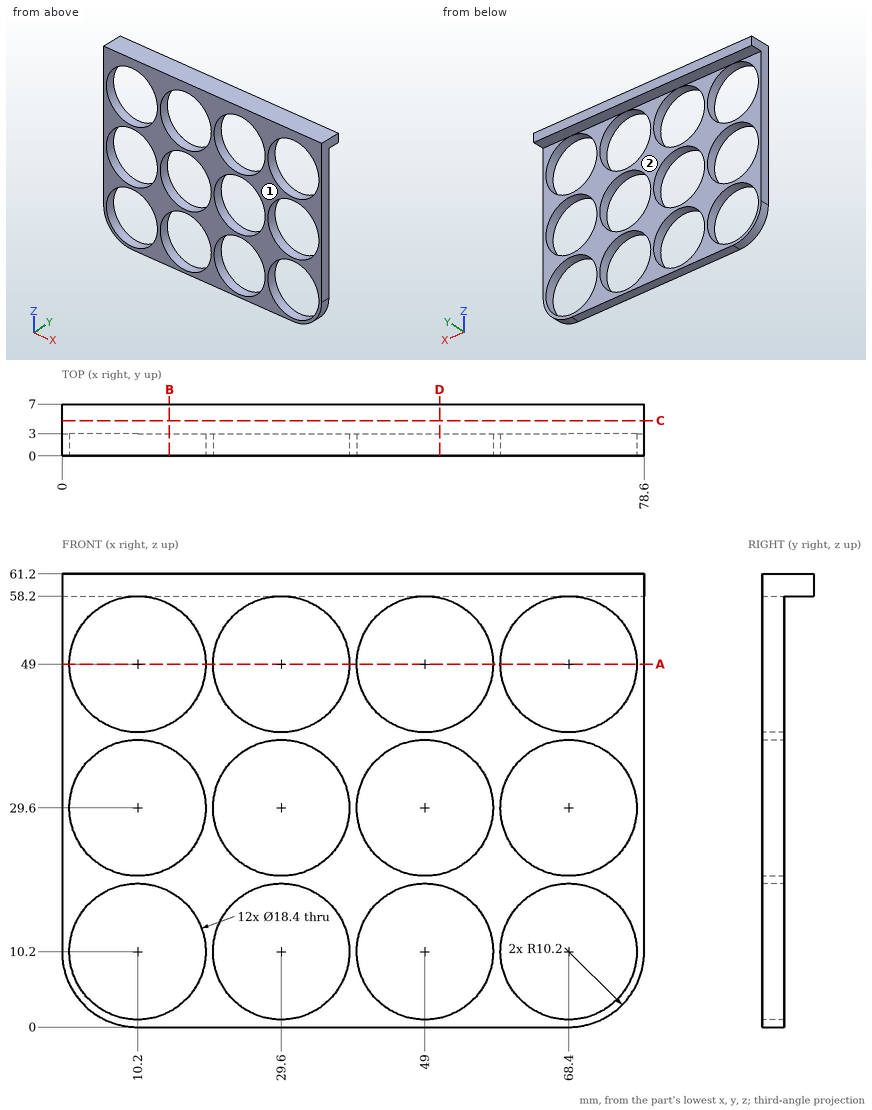
The drawing under review shows one solid part. Ordinate dimensions are in mm from its lowest x, y, z. A direction names the side the tool comes from. Give positions to 0.01 mm unless a question says otherwise; leave off trailing zeros. Order: outer loops, then holes, each group sorted by start corner. A loop starts at its lowest first (then second) coordinate and runs counter-clockwise, first axis right, second up. Notation, with made-up numbers: M 80.25,76 L 110.25,76 A21 ccw 110.25,83 Z; hole C -21,54.5 d8. An arc over 180 degrees is marked long. Answer in a Markdown table with one row per item. Add a question column.
1. Add section D-D on x = 51. State the section outline as (y, z) points.
2. For pin 1 Ø24 at (x, z) = (29.6, 10.2) entering from +Y; pin 2 Ø16.5 at (x, z) = (49, 29.6) entering from +Y; pin 3 Ø1.2 at (x, y) = (29.5, 6) entering from -Z, all flat-tipped, find the tip position at first contact; note any pin that passes through.
3. To check wall thickness, follow line 1 along X through (y, z) = (1.55, 29.6); line 2 along Z through (x, y) = (50, 2.5); line 3 along Z through (x, y) = (16, 4.5). State the ranges of each line that lie inside material, in increasing order.
4. Add section C-C on y = 4.75. State the section outline as (x, z) points, plus the area to 3 significant figures.
5. Machinability: for the marked faces 1 and 2, which of the approach directions +Z, -Z, +X, -X, +Y, -Y give a long, thin tool a straight path to every point of the face, cutting with its end or side? Answer none if there is none.
6. Add section B-B on x = 14.5. State the section outline as (y, z) points, plus the area to 3 significant figures.
7. Add section A-A on z = 49. State the section outline as (x, y) points.
The answers:
| question | item | result |
|---|---|---|
| 1 | outline | M 0,0 L 3,0 L 3,1.22 L 0,1.22 Z; M 0,19.18 L 3,19.18 L 3,20.62 L 0,20.62 Z; M 0,38.58 L 3,38.58 L 3,40.02 L 0,40.02 Z; M 0,57.98 L 3,57.98 L 3,58.2 L 7,58.2 L 7,61.2 L 0,61.2 Z |
| 2 | pin 1 | y = 3 |
| 2 | pin 2 | through |
| 2 | pin 3 | z = 58.2 |
| 3 | line 1 | 0 to 1, 19.4 to 20.4, 38.8 to 39.8, 58.2 to 59.2, 77.6 to 78.6 |
| 3 | line 2 | 0 to 1.05, 19.35 to 20.45, 38.75 to 39.85, 58.15 to 61.2 |
| 3 | line 3 | 58.2 to 61.2 |
| 4 | outline | M 0,58.2 L 78.6,58.2 L 78.6,61.2 L 0,61.2 Z |
| 4 | area | 236 mm2 |
| 5 | face 1 | +Z, -Z, +X, -X, -Y |
| 5 | face 2 | -Z, +X, -X, +Y |
| 6 | outline | M 0,0 L 3,0 L 3,2.07 L 0,2.07 Z; M 0,18.33 L 3,18.33 L 3,21.47 L 0,21.47 Z; M 0,37.73 L 3,37.73 L 3,40.87 L 0,40.87 Z; M 0,57.13 L 3,57.13 L 3,58.2 L 7,58.2 L 7,61.2 L 0,61.2 Z |
| 6 | area | 49.2 mm2 |
| 7 | outline | M 0,0 L 1,0 L 1,3 L 0,3 Z; M 19.4,0 L 20.4,0 L 20.4,3 L 19.4,3 Z; M 38.8,0 L 39.8,0 L 39.8,3 L 38.8,3 Z; M 58.2,0 L 59.2,0 L 59.2,3 L 58.2,3 Z; M 77.6,0 L 78.6,0 L 78.6,3 L 77.6,3 Z |
